Read the model definition and answer for the solid it produces. Units are mm, in the model's axes. A direction names the side the tool comes from. Round coordinates to 2 decimals unless told otherwise and drop trailing zeros. Loops run counter-clockwise (first coordinate to the right, second up) from the corner with the lowest first, then second, coordinate; pieces in that order, holes last. Notation, with made-up numbers: (2, 1) -> (12, 1) arc R36 ccw to (12, 36) -> close; hole circle Ø11 at (-28.75, 72). An arc over 180 degrees is marked (long way). Put each result on its own line as item: value.
from build123d import *

# Parameters (mm, degrees)
PAD_DEPTH    = 9
SKETCH001_R  = 4.1
PAD001_DEPTH = 1.5
SKETCH002_R  = 4
PAD002_DEPTH = 7
PAD003_DEPTH = 1.5
PAD004_DEPTH = 7
SKETCH005_R  = 1.5
POCKET_DEPTH = 17.501
CHAMFER_SIZE = 0.5


with BuildPart() as part:
    # Sketch → Pad (new body)
    with BuildSketch(Plane.XY):
        Polygon((-59.96273, 0.078839), (36.03727, 0.078839), (36.03727, 14.078839), (7.03727, 14.078839), (7.03727, 9.078839), (-59.96273, 9.078839), align=None)
    extrude(amount=PAD_DEPTH)

    # Sketch001 → Pad001 (new body)
    with BuildSketch(Plane.XY.offset(9)):
        with Locations((22.03727, 8.078839)):
            Circle(SKETCH001_R)
    extrude(amount=PAD001_DEPTH)

    # Sketch002 → Pad002 (new body)
    with BuildSketch(Plane.XY.offset(10.5)):
        with Locations((22.03727, 8.078839)):
            Circle(SKETCH002_R)
    extrude(amount=PAD002_DEPTH)

    # Sketch003 → Pad003 (new body)
    with BuildSketch(Plane.XZ.offset(-0.078839)):
        with BuildLine():
            ThreePointArc((-15.96499, 0), (-18.96273, 6.897062), (-21.960469, 0))
            Line((-21.960469, 0), (-15.96499, 0))
        make_face()
    extrude(amount=PAD003_DEPTH)

    # Sketch004 → Pad004 (new body)
    with BuildSketch(Plane.XZ.offset(1.421161)):
        with BuildLine():
            ThreePointArc((-16.103281, 0), (-18.96273, 6.797062), (-21.822178, 0))
            Line((-21.822178, 0), (-16.103281, 0))
        make_face()
    extrude(amount=PAD004_DEPTH)

    # Sketch005 → Pocket (cut, through all)
    with BuildSketch(Plane(origin=(0, 9.078839, 0), x_dir=(-1, 0, 0), z_dir=(0, 1, 0))):
        with Locations((55.46273, 4.5)):
            Circle(SKETCH005_R)
    extrude(amount=-POCKET_DEPTH, mode=Mode.SUBTRACT)

    # Chamfer
    chamfer_edges = [part.edges().sort_by_distance(p)[0] for p in [
        (-18.96273, -8.421161, 6.797062),
        (18.03727, 8.078839, 17.5),
    ]]
    chamfer(chamfer_edges, length=CHAMFER_SIZE)


solid = part.part
Item 1: Find the intervals of material crossed by line 1 along Z through (x, y) = (16, 5); line 2 along Y through (x, z) = (-20, 8.75); line 3 along Y through (x, z) = (19, 8.5), in increasing order.
Derived:
line 1: z = 0 to 9
line 2: y = 0.08 to 9.08
line 3: y = 0.08 to 14.08
Item 2: Which of the six approach directions +Z, -Z, +X, -X, +Y, -Y give full straight-line access (tool end or side, diameter ignored) to faces 5 (the flat face through (36.037, 7, 4)), 6 (the cylindrical face through (-18.829, -0.661, 6.895)), 7 (the flat face through (7.037, 12, 4)), 8 (the cylindrical face through (18.04, 8.25, 13.7)), 9 (the flat face through (22, 8, 17.5))?
Derived:
face 5: +Z, -Z, +X, +Y, -Y
face 6: -Y
face 7: +Z, -Z, -X, +Y
face 8: +Z
face 9: +Z, +X, -X, +Y, -Y
Item 3: For a pull along Z with two mould halves and no side action, classify faces 1 (the flat face through (-26, 9.079, 4)), 2 (the flat face through (-13, 5, 0)), 3 (the cylindrical face through (-18.831, -4.626, 6.795)), 4 (the cylindrical face through (-54.27, 4.64, 3.59)) as pulls with the +Z half, pulls with the -Z half, needs draft (parallel to the pull), parting line crosses it, or undercut.
Derived:
face 1: needs draft
face 2: pulls with the -Z half
face 3: parting line crosses it
face 4: undercut
Item 4: The part is cut by section A-A (y = 1.75). Determine the outline of the cut face in (x, z), then the cut area to 3 significant figures.
Derived:
outline: (-59.96, 0) -> (36.04, 0) -> (36.04, 9) -> (-59.96, 9) -> close; hole circle Ø3 at (-55.46, 4.5)
area: 857 mm^2
Item 5: Flat-ended cylindrical pins translate along their axes: pin 1 Ø10 at (x, z) = (-34.5, 4) entering from +Y; pin 2 Ø10 at (y, z) = (9.5, 15) entering from -X; pin 3 Ø3 at (x, y) = (1, -0.5) entering from +Z. Find the tip coordinate at first contact, or state that the pin passes through.
Derived:
pin 1: stops at y = 9.08
pin 2: stops at x = 17.94
pin 3: stops at z = 9
Item 6: The part is cut by section C-C (y = -4.25). Determine the outline of the cut face in (x, z).
Derived:
outline: (-21.82, 0) -> (-16.1, 0) arc R4 ccw (long way) to start
Item 7: The part is cut by section B-B (z = 15.5). Determine the outline of the cut face in (x, y), then the cut area to 3 significant figures.
Derived:
outline: circle Ø8 at (22.04, 8.08)
area: 50.3 mm^2
